Geometry: final body of the model. Coordinates: model frame, mm. Face numbers are marked on the shaded views. A direction names the side the tool comes from. Give positions to 0.01 mm unless a question says otherwise; leave off trailing zeros. Write each loop counter-clockwise with the first axis right and the second up, starting at its lowest first coordinate (ties: lowest second). Pieces come first, ordered by that corner, then holes. Notation, with made-up numbers: M -9.5,42.25 L 21.5,42.25 A6 ccw 21.5,53.25 Z; hole C 65.25,15.25 d11. An arc over 180 degrees is marked long. Answer as a JSON object with one key per item and string values.
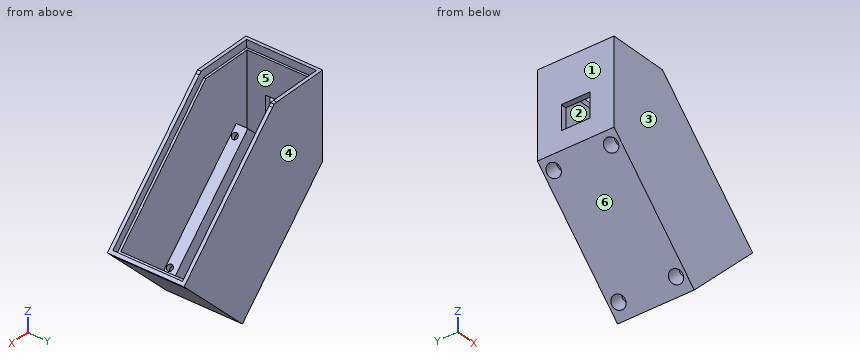
from build123d import *

# Parameters (mm, degrees)
BOSS_EXTRUDE1_DEPTH = 40
SHELL1_T            = -3
BOSS_EXTRUDE2_DEPTH = 4
BOSS_EXTRUDE3_DEPTH = 4
BOSS_EXTRUDE4_DEPTH = 1.8
BOSS_EXTRUDE5_DEPTH = 1.8
SKETCH10_R          = 1.65
CUT_EXTRUDE6_DEPTH  = 41.105
SKETCH11_W          = 12.8
SKETCH11_H          = 15
CUT_EXTRUDE7_DEPTH  = 3
SKETCH12_W          = 69.967359313
SKETCH12_H          = 34
SKETCH12_R          = 1.6
BOSS_EXTRUDE7_DEPTH = 10
SKETCH13_R          = 3.5
CUT_EXTRUDE9_DEPTH  = 10
SKETCH14_W          = 69.967359313
SKETCH14_H          = 22
CUT_EXTRUDE10_DEPTH = 10


with BuildPart() as part:
    # Sketch1 → Boss-Extrude1 (new body)
    with BuildSketch(Plane(origin=(0, 0, 0), x_dir=(1, 0, 0), z_dir=(0, 1, 0))):
        Polygon((-43.359374855, -5.394325428), (-43.359374855, 35.316352691), (9.115019377, 87.790746923), (44.470358437, 52.435407864), (-13.359374855, -5.394325428), align=None)
    extrude(amount=BOSS_EXTRUDE1_DEPTH)

    # Shell1
    shell1_openings = [part.faces().sort_by_distance(p)[0] for p in [
        (15.555491791, 20, -23.520541218),
        (-28.359374855, 20, 5.394325428),
    ]]
    offset(amount=SHELL1_T, openings=shell1_openings, kind=Kind.INTERSECTION)

    # Sketch6 → Boss-Extrude2 (add)
    with BuildSketch(Plane(origin=(-3.982524714, 0, -3.982524714), x_dir=(0.707106781, 0, -0.707106781), z_dir=(0.707106781, 0, 0.707106781))):
        Polygon((-13.260868642, 38.2), (66.722724487, 38.2), (66.722724487, 1.8), (-13.260868642, 1.8), (-13.260868642, 0), (68.522724487, 0), (68.522724487, 40), (-13.260868642, 40), align=None)
    extrude(amount=BOSS_EXTRUDE2_DEPTH)

    # Sketch7 → Boss-Extrude3 (add)
    with BuildSketch(Plane.XY.offset(5.394325428)):
        Polygon((-13.359374855, 1.8), (-41.559374855, 1.8), (-41.559374855, 38.2), (-13.359374855, 38.2), (-13.359374855, 40), (-43.359374855, 40), (-43.359374855, 0), (-13.359374855, 0), align=None)
    extrude(amount=BOSS_EXTRUDE3_DEPTH)

    # Sketch8 → Boss-Extrude4 (add)
    with BuildSketch(Plane.XZ):
        Polygon((-13.359374855, 9.394325428), (-11.702520605, 9.394325428), (-10.53094773, 8.222752552), (-13.359374855, 5.394325428), align=None)
    extrude(amount=-BOSS_EXTRUDE4_DEPTH)

    # Sketch9 → Boss-Extrude5 (add)
    with BuildSketch(Plane(origin=(0, 40, 0), x_dir=(1, 0, 0), z_dir=(0, 1, 0))):
        Polygon((-13.359374855, -5.394325428), (-10.53094773, -8.222752552), (-11.553745116, -9.245549939), (-13.359374855, -9.394325428), align=None)
    extrude(amount=-BOSS_EXTRUDE5_DEPTH)

    # Sketch10 → Cut-Extrude6 (cut, through all)
    with BuildSketch(Plane(origin=(-37.216543429, 0, -37.216543429), x_dir=(0.707106781, 0, -0.707106781), z_dir=(0.707106781, 0, 0.707106781))):
        with Locations((60.522724487, 35)):
            Circle(SKETCH10_R)
        with Locations((60.522724487, 5)):
            Circle(SKETCH10_R)
        with Locations((0.522724487, 35)):
            Circle(SKETCH10_R)
        with Locations((0.522724487, 5)):
            Circle(SKETCH10_R)
    extrude(amount=-CUT_EXTRUDE6_DEPTH, mode=Mode.SUBTRACT)

    # Sketch11 → Cut-Extrude7 (cut)
    with BuildSketch(Plane(origin=(-40.359374855, 0, 0), x_dir=(0, 0, -1), z_dir=(1, 0, 0))):
        with Locations((19.207640819, 20)):
            Rectangle(SKETCH11_W, SKETCH11_H)
    extrude(amount=-CUT_EXTRUDE7_DEPTH, mode=Mode.SUBTRACT)

    # Sketch12 → Boss-Extrude7 (add)
    with BuildSketch(Plane(origin=(-37.216543429, 0, -37.216543429), x_dir=(0.707106781, 0, -0.707106781), z_dir=(0.707106781, 0, 0.707106781))):
        with Locations((30.539044831, 20)):
            Rectangle(SKETCH12_W, SKETCH12_H)
        with Locations((0.522724487, 35)):
            Circle(SKETCH12_R, mode=Mode.SUBTRACT)
        with Locations((60.522724487, 35)):
            Circle(SKETCH12_R, mode=Mode.SUBTRACT)
        with Locations((60.522724487, 5)):
            Circle(SKETCH12_R, mode=Mode.SUBTRACT)
        with Locations((0.522724487, 5)):
            Circle(SKETCH12_R, mode=Mode.SUBTRACT)
    extrude(amount=BOSS_EXTRUDE7_DEPTH)

    # Sketch13 → Cut-Extrude9 (cut)
    with BuildSketch(Plane(origin=(-39.337863773, 0, -39.337863773), x_dir=(-0.707106781, 0, 0.707106781), z_dir=(-0.707106781, 0, -0.707106781))):
        with Locations((-0.522724487, 35)):
            Circle(SKETCH13_R)
        with Locations((-0.522724487, 5)):
            Circle(SKETCH13_R)
        with Locations((-60.522724487, 5)):
            Circle(SKETCH13_R)
        with Locations((-60.522724487, 35)):
            Circle(SKETCH13_R)
    extrude(amount=-CUT_EXTRUDE9_DEPTH, mode=Mode.SUBTRACT)

    # Sketch14 → Cut-Extrude10 (cut)
    with BuildSketch(Plane(origin=(-30.145475617, 0, -30.145475617), x_dir=(0.707106781, 0, -0.707106781), z_dir=(0.707106781, 0, 0.707106781))):
        with Locations((30.539044831, 20)):
            Rectangle(SKETCH14_W, SKETCH14_H)
    extrude(amount=-CUT_EXTRUDE10_DEPTH, mode=Mode.SUBTRACT)


solid = part.part
1) Contact query for flat-ended pins moving along their axis: P1, Ø17, axis at x = -8.5, z = -59, coming from the -Y side; P2, Ø10, axis at y = 5.5, z = -47, coming from the +X side; P3, Ø2.5, axis at x = -42, y = 18.5, coming from the -Z side; P4, Ø5, axis at y = 13, z = -63.5, coming from the +X side. Output: stop coordinate, or through.
Geometry check:
{"P1": "stops at y = 0", "P2": "stops at x = 47.3", "P3": "stops at z = -37.93", "P4": "stops at x = 35.91"}
2) Pull-direction query (Y, two-part tool) for the marked faces 3, 4, 5 and 6; classes: pulls with the +Y half, pulls with the -Y half, needs draft (parallel to the pull), parting line crosses it, or undercut.
Geometry check:
{"face 3": "pulls with the -Y half", "face 4": "pulls with the +Y half", "face 5": "undercut", "face 6": "needs draft"}
3) Cut plane C-C on x = -20.5. Return loops of the section in (y, z), and give its area (3 significant figures).
Geometry check:
{"outline": "M 0,-58.18 L 40,-58.18 L 40,9.39 L 38.2,9.39 L 38.2,5.39 L 37,5.39 L 37,-39.79 L 31,-39.79 L 31,-53.93 L 9,-53.93 L 9,-39.79 L 3,-39.79 L 3,5.39 L 1.8,5.39 L 1.8,9.39 L 0,9.39 Z", "area": "710 mm2"}
4) Set-up query: the marked faces 1 and 2. Return all of +Z, -Z, +X, -X, +Y, -Y with unobstructed straight access to the full face (end or side cutting, diameter ignored); none if empty.
Geometry check:
{"face 1": "+Z, -Z, -X, +Y, -Y", "face 2": "+Z"}
5) Cut plane A-A on y = 24. Return loops of the section in (x, z).
Geometry check:
{"outline": "M -43.36,-35.32 L 9.12,-87.79 L 47.3,-49.61 L 46.03,-48.33 L 43.2,-51.16 L 42.35,-50.31 L 9.12,-83.55 L -40.36,-34.07 L -40.36,-25.61 L -43.36,-25.61 Z; M -43.36,-12.81 L -40.36,-12.81 L -40.36,5.39 L -41.56,5.39 L -41.56,9.39 L -43.36,9.39 Z"}
6) Line query: line 1 (Y direction, x = -7.5, z = -25.5); line 2 (Y direction, x = -4, z = -2.5); line 3 (X direction, y = 14, z = -30.5). Output: solid intervals per line, ascending. Write a range as from..to.
Geometry check:
{"line 1": "y = 0..3, 37..40", "line 2": "y = 0..1.8, 38.2..40", "line 3": "x = -43.36..-40.36"}
7) Cut plane D-D on z = -46. Return loops of the section in (x, y), and give its area (3 significant figures).
Geometry check:
{"outline": "M -32.68,0 L 43.69,0 L 43.69,1.8 L 38.03,1.8 L 38.03,3 L -14.29,3 L -14.29,9 L -28.43,9 L -28.43,31 L -14.29,31 L -14.29,37 L 38.03,37 L 38.03,38.2 L 43.69,38.2 L 43.69,40 L -32.68,40 Z", "area": "759 mm2"}
8) Cut plane B-B on z = -60.5. Return loops of the section in (x, y), and give its area (3 significant figures).
Geometry check:
{"outline": "M -18.18,0 L 36.41,0 L 36.41,40 L -18.18,40 Z; hole M -13.93,9 L 0.21,9 L 0.21,3 L 32.16,3 L 32.16,37 L 0.21,37 L 0.21,31 L -13.93,31 Z", "area": "786 mm2"}
